Autodesk Inventor part; units mm, degrees
ref_plane "ANBAU_1_XY" through (0, 0, -21) normal (0, 0, 1) x (1, 0, 0)
ref_plane "ANBAU_1_YZ" through (0, 0, -21) normal (1, 0, 0) x (0, 1, 0)
ref_plane "ANBAU_1_ZX" through (0, 0, -21) normal (0, 1, 0) x (0, 0, 1)
sketch "Sketch_1" plane through (0, 0, 0) normal (0, 0, 1) x (1, 0, 0)
  arc A0 (-29.9895, 25.2782) -> (-29.9895, -25.2782) centre (419.3, 0) ccw
  arc A1 (-29.9895, -25.2782) -> (-25.2782, -29.9895) centre (-24.9973, -24.9973) ccw
  arc A2 (-25.2782, -29.9895) -> (25.2782, -29.9895) centre (0, 419.3) ccw
  arc A3 (25.2782, -29.9895) -> (29.9895, -25.2782) centre (24.9973, -24.9973) ccw
  arc A4 (29.9895, -25.2782) -> (29.9895, 25.2782) centre (-419.3, 0) ccw
  arc A5 (29.9895, 25.2782) -> (25.2782, 29.9895) centre (24.9973, 24.9973) ccw
  arc A6 (25.2782, 29.9895) -> (-25.2782, 29.9895) centre (0, -419.3) ccw
  arc A7 (-25.2782, 29.9895) -> (-29.9895, 25.2782) centre (-24.9973, 24.9973) ccw
  circle A8 centre (19, 0) radius 2.25
  circle A9 centre (0, 19) radius 2.25
  circle A10 centre (0, -19) radius 2.25
  circle A11 centre (-19, 0) radius 2.25
extrude "Extrusion1" add sketch "Sketch_1" against normal blind 21
sketch "Sketch_2" plane through (0, 0, 0) normal (1, 0, 0) x (0, 1, 0)
  line L0 (0, -21) -> (0, 0)
  line L1 (0, 0) -> (25.2887, 0)
  line L2 (25.2887, 0) -> (25, -0.5)
  line L3 (25, -0.5) -> (25, -3.7)
  arc A0 (24.7, -4) -> (25, -3.7) centre (24.7, -3.7) ccw
  line L4 (24.7, -4) -> (16, -4)
  line L5 (16, -4) -> (16, -18.7)
  line L6 (16, -18.7) -> (21.7, -18.7)
  arc A1 (22, -19) -> (21.7, -18.7) centre (21.7, -19) ccw
  line L7 (22, -19) -> (22, -20.5)
  line L8 (22, -20.5) -> (22.2887, -21)
  line L9 (22.2887, -21) -> (0, -21)
  line L10 (0, -21) -> (0, 0)
revolve "Revolution1" cut sketch "Sketch_2" angle 360 about axis through (0, 0, -21) along (0, 0, -1)
sketch "Sketch_3" plane through (0, 0, 0) normal (0, 0, 1) x (1, 0, 0)
  arc A0 (-19, 4) -> (-19, -4) centre (-19, 0) ccw
  line L0 (-19, -4) -> (-4, -4)
  line L1 (-4, -4) -> (-4, -19)
  arc A1 (-4, -19) -> (4, -19) centre (0, -19) ccw
  line L2 (4, -19) -> (4, -4)
  line L3 (4, -4) -> (19, -4)
  arc A2 (19, -4) -> (19, 4) centre (19, 0) ccw
  line L4 (19, 4) -> (4, 4)
  line L5 (4, 4) -> (4, 19)
  arc A3 (4, 19) -> (-4, 19) centre (0, 19) ccw
  line L6 (-4, 19) -> (-4, 4)
  line L7 (-4, 4) -> (-19, 4)
extrude "Extrusion2" cut sketch "Sketch_3" against normal blind 8
sketch "Sketch4" plane through (0, 0, 0) normal (0, 0, 1) x (1, 0, 0)
  point P0 (24.7487, 24.7487)
hole "Hole1" at (24.7487, 24.7487, 0) direction (0, 0, -1) diameter 3.242 depth 12.2188 tip angle 120 countersink diameter 4 countersink angle 90
sketch "Sketch5" plane through (0, 0, 0) normal (0, 0, 1) x (1, 0, 0)
  point P0 (-24.7487, -24.7487)
hole "Hole2" at (-24.7487, -24.7487, 0) direction (0, 0, -1) diameter 3.242 depth 12.2188 tip angle 120 countersink diameter 4 countersink angle 90
sketch "Sketch6" plane through (0, 0, 0) normal (0, 0, 1) x (1, 0, 0)
  point P0 (24.7487, -24.7487)
hole "Hole3" at (24.7487, -24.7487, 0) direction (0, 0, -1) diameter 3.242 depth 12.2188 tip angle 120 countersink diameter 4 countersink angle 90
sketch "Sketch7" plane through (0, 0, 0) normal (0, 0, 1) x (1, 0, 0)
  point P0 (-24.7487, 24.7487)
hole "Hole4" at (-24.7487, 24.7487, 0) direction (0, 0, -1) diameter 3.242 depth 12.2188 tip angle 120 countersink diameter 4 countersink angle 90
ref_plane "ANBAU_1_XY" through (0, 0, -21) normal (0, 0, 1) x (1, 0, 0)
ref_plane "ANBAU_1_YZ" through (0, 0, -21) normal (1, 0, 0) x (0, 1, 0)
ref_plane "ANBAU_1_ZX" through (0, 0, -21) normal (0, 1, 0) x (0, 0, 1)
ref_plane "ZYL_SCHRAUBE_1_1_XY" through (24.7487, 24.7487, 9) normal (0, 0, -1) x (1, 0, 0)
ref_plane "ZYL_SCHRAUBE_1_1_YZ" through (24.7487, 24.7487, 9) normal (1, 0, 0) x (0, -1, 0)
ref_plane "ZYL_SCHRAUBE_1_1_ZX" through (24.7487, 24.7487, 9) normal (0, -1, 0) x (0, 0, -1)
ref_plane "ZYL_SCHRAUBE_1_2_XY" through (-24.7487, 24.7487, 9) normal (0, 0, -1) x (1, 0, 0)
ref_plane "ZYL_SCHRAUBE_1_2_YZ" through (-24.7487, 24.7487, 9) normal (1, 0, 0) x (0, -1, 0)
ref_plane "ZYL_SCHRAUBE_1_2_ZX" through (-24.7487, 24.7487, 9) normal (0, -1, 0) x (0, 0, -1)
ref_plane "ZYL_SCHRAUBE_1_3_XY" through (-24.7487, -24.7487, 9) normal (0, 0, -1) x (1, 0, 0)
ref_plane "ZYL_SCHRAUBE_1_3_YZ" through (-24.7487, -24.7487, 9) normal (1, 0, 0) x (0, -1, 0)
ref_plane "ZYL_SCHRAUBE_1_3_ZX" through (-24.7487, -24.7487, 9) normal (0, -1, 0) x (0, 0, -1)
ref_plane "ZYL_SCHRAUBE_1_4_XY" through (24.7487, -24.7487, 9) normal (0, 0, -1) x (1, 0, 0)
ref_plane "ZYL_SCHRAUBE_1_4_YZ" through (24.7487, -24.7487, 9) normal (1, 0, 0) x (0, -1, 0)
ref_plane "ZYL_SCHRAUBE_1_4_ZX" through (24.7487, -24.7487, 9) normal (0, -1, 0) x (0, 0, -1)
ref_plane "ZYL_SCHRAUBE_2_1_XY" through (19, 0, -8) normal (0, 0, -1) x (1, 0, 0)
ref_plane "ZYL_SCHRAUBE_2_1_YZ" through (19, 0, -8) normal (1, 0, 0) x (0, -1, 0)
ref_plane "ZYL_SCHRAUBE_2_1_ZX" through (19, 0, -8) normal (0, -1, 0) x (0, 0, -1)
ref_plane "ZYL_SCHRAUBE_2_2_XY" through (0, 19, -8) normal (0, 0, -1) x (1, 0, 0)
ref_plane "ZYL_SCHRAUBE_2_2_YZ" through (0, 19, -8) normal (1, 0, 0) x (0, -1, 0)
ref_plane "ZYL_SCHRAUBE_2_2_ZX" through (0, 19, -8) normal (0, -1, 0) x (0, 0, -1)
ref_plane "ZYL_SCHRAUBE_2_3_XY" through (-19, 0, -8) normal (0, 0, -1) x (1, 0, 0)
ref_plane "ZYL_SCHRAUBE_2_3_YZ" through (-19, 0, -8) normal (1, 0, 0) x (0, -1, 0)
ref_plane "ZYL_SCHRAUBE_2_3_ZX" through (-19, 0, -8) normal (0, -1, 0) x (0, 0, -1)
ref_plane "ZYL_SCHRAUBE_2_4_XY" through (0, -19, -8) normal (0, 0, -1) x (1, 0, 0)
ref_plane "ZYL_SCHRAUBE_2_4_YZ" through (0, -19, -8) normal (1, 0, 0) x (0, -1, 0)
ref_plane "ZYL_SCHRAUBE_2_4_ZX" through (0, -19, -8) normal (0, -1, 0) x (0, 0, -1)
properties part number "1956846 EAMF-A-44C-60P(1A10)"
Source: CAD feature listing. Evaluate the final solid. Frame: model axes, mm. A direction names the side the tool comes from. Round coordinates to 2 decimals unless told otherwise and drop trailing zeros. Loops run counter-clockwise (first coordinate to the right, second up) from the corner with the lowest first, then second, coordinate; pieces in that order, holes last. Notation, with made-up numbers: (23.25, -22) - (73.25, -22) arc R11 cw to (73.25, -3) - close; hole circle Ø1 at (81, 72.25). An arc over 180 degrees is marked (long way). Write item = value, one per line. Start each with the question number.
Item 1: Material intervals for line 1 (Y direction, x = 0, z = -13); line 2 (X direction, y = 0, z = -1.85); line 3 (X direction, y = 0, z = -19.4), sorted ascending.
Item 2: Section query D-D on z = -5.25. Output: boundary loops of the cut face in (x, y), plus the area to 3 significant figures.
Item 3: First-contact query: pin 1 Ø5 at (x, y) = (0.5, 12) entering from +Z; pin 2 Ø4 at (y, z) = (1, -9) entering from -X; pin 3 Ø1.1 at (y, z) = (18, -5.5) entering from -X; pin 4 Ø4 at (x, z) = (-17.5, -5) entering from +Y. Flat tips, straight axial feed; report the tip coordinate or a pass-through.
Item 4: Section query A-A on z = -16.5. Output: boundary loops of the cut face in (x, y).
Item 5: Reachability of faces 5 (the face through (-13, -10, -18.7)), 6 (the face through (2, -21, -8)), 7 (the face through (-6.13, 14.78, -11.45)) from +Z, -Z, +X, -X, +Y, -Y: full face, straight path, thin tool, end or side. Return the list, or none.
Item 6: Section query B-B on z = -10.5. Count the separate pieces of the cut face and the enclosed holes in it, plus the area to 3 significant figures.
Item 7: Mould query, pull axis Y, two halves, no side actions, for faces 1 (the face through (-0.488, 16.804, -13.275)), 2 (the face through (26.187, -25.497, -6.382)), 3 (the face through (-30.7, 0.4, -10.4)), 4 (the face through (13, 21, -21)). Classes: released by +Y, released by -Y, zero draft, split by the parting line, or undercut.
Results list:
q1.line_1 = -30.7 to -21.25, -16.75 to -16, 16 to 16.75, 21.25 to 30.7
q1.line_2 = -30.7 to -25, 25 to 30.7
q1.line_3 = -30.7 to -22, 22 to 30.7
q2.outline = (-29.99, -25.28) arc R5 ccw to (-25.28, -29.99) arc R450 ccw to (25.28, -29.99) arc R5 ccw to (29.99, -25.28) arc R450 ccw to (29.99, 25.28) arc R5 ccw to (25.28, 29.99) arc R450 ccw to (-25.28, 29.99) arc R5 ccw to (-29.99, 25.28) arc R450 ccw to start; hole circle Ø3.24 at (-24.75, -24.75); hole circle Ø3.24 at (-24.75, 24.75); hole (-19, -4) - (-15.49, -4) arc R16 ccw to (-4, -15.49) - (-4, -19) arc R4 ccw to (4, -19) - (4, -15.49) arc R16 ccw to (15.49, -4) - (19, -4) arc R4 ccw to (19, 4) - (15.49, 4) arc R16 ccw to (4, 15.49) - (4, 19) arc R4 ccw to (-4, 19) - (-4, 15.49) arc R16 ccw to (-15.49, 4) - (-19, 4) arc R4 ccw to start; hole circle Ø3.24 at (24.75, -24.75); hole circle Ø3.24 at (24.75, 24.75)
q2.area = 2,630 mm²
q3.pin_1 = through
q3.pin_2 = -30.7
q3.pin_3 = -30.36
q3.pin_4 = 30.43
q4.outline = (-29.99, -25.28) arc R5 ccw to (-25.28, -29.99) arc R450 ccw to (25.28, -29.99) arc R5 ccw to (29.99, -25.28) arc R450 ccw to (29.99, 25.28) arc R5 ccw to (25.28, 29.99) arc R450 ccw to (-25.28, 29.99) arc R5 ccw to (-29.99, 25.28) arc R450 ccw to start; hole circle Ø4.5 at (-19, 0); hole circle Ø32 at (0, 0); hole circle Ø4.5 at (0, -19); hole circle Ø4.5 at (0, 19); hole circle Ø4.5 at (19, 0)
q5.face_5 = -Z
q5.face_6 = +Z
q5.face_7 = +Z, -Z
q6.separate_pieces = 1
q6.enclosed_holes = 9
q6.area = 2,770 mm²
q7.face_1 = undercut
q7.face_2 = undercut
q7.face_3 = split by the parting line
q7.face_4 = zero draft
